The listing builds one solid part. Answer for the finished solid, in the listing's coordinates (mm). A direction names the side the tool comes from. Round coordinates to 2 decimals unless told otherwise and drop trailing zeros. Order: outer loops, then holes, each group sorted by start corner. A loop starts at its lowest first (then second) coordinate and runs counter-clockwise, first axis right, second up. Notation, with made-up numbers: (56.5, 55) - (111.5, 55) arc R13 ccw to (111.5, 65) - close; hole circle Ø4 at (68.25, 72.5). An arc over 180 degrees is marked (long way). Write item = value, one per line.
from build123d import *

# Parameters (mm, degrees)
BOSS_EXTRUDE1_DEPTH = 3.175


with BuildPart() as part:
    # Sketch1 → Boss-Extrude1 (new, symmetric)
    with BuildSketch(Plane.XY):
        with BuildLine():
            Line((-54.61, -57.15), (54.61, -57.15))
            ThreePointArc((54.61, -57.15), (56.406051224, -56.406051224), (57.15, -54.61))
            Line((57.15, -54.61), (57.15, 54.61))
            ThreePointArc((57.15, 54.61), (56.406051224, 56.406051224), (54.61, 57.15))
            Line((54.61, 57.15), (-54.61, 57.15))
            ThreePointArc((-54.61, 57.15), (-56.406051224, 56.406051224), (-57.15, 54.61))
            Line((-57.15, 54.61), (-57.15, -54.61))
            ThreePointArc((-57.15, -54.61), (-56.406051224, -56.406051224), (-54.61, -57.15))
        make_face()
        with BuildLine():
            Line((-45.72, -48.26), (11.649731947, -48.26))
            Line((11.649731947, -48.26), (45.72, -48.26))
            ThreePointArc((45.72, -48.26), (47.516051224, -47.516051224), (48.26, -45.72))
            Line((48.26, -45.72), (48.26, -17.513600374))
            Line((48.26, -17.513600374), (48.26, 45.72))
            ThreePointArc((48.26, 45.72), (47.516051224, 47.516051224), (45.72, 48.26))
            Line((45.72, 48.26), (12.317525133, 48.26))
            Line((12.317525133, 48.26), (-45.9238932, 48.26))
            ThreePointArc((-45.9238932, 48.26), (-46.572550677, 48.344222429), (-47.178191218, 48.591304348))
            ThreePointArc((-47.178191218, 48.591304348), (-54.010842502, 46.063523076), (-50.35826087, 39.760075674))
            ThreePointArc((-50.35826087, 39.760075674), (-48.854027571, 38.891201551), (-48.26, 37.2587827))
            Line((-48.26, 37.2587827), (-48.26, -0.752095073))
            Line((-48.26, -0.752095073), (-48.26, -45.72))
            ThreePointArc((-48.26, -45.72), (-47.516051224, -47.516051224), (-45.72, -48.26))
        make_face(mode=Mode.SUBTRACT)
    extrude(amount=BOSS_EXTRUDE1_DEPTH, both=True)


solid = part.part
Q1. Determine the mould class of faces 3 (the face through (-47.536, -47.496, 0.044)), 4 (the face through (-1, -57.15, 0)), 5 (the face through (-56.426, -56.386, 0.044)) for opening direction X: released by +X, released by -X, zero draft, split by the parting line, or undercut.
Model answer:
face_3 = undercut
face_4 = zero draft
face_5 = released by -X
Q2. Section A-A on x = -30.5 is taken. Determine the outline of the cut face in (y, z) (3 decimals), then the cut area to 3 significant figures.
Model answer:
outline = (-57.15, -3.175) - (-48.26, -3.175) - (-48.26, 3.175) - (-57.15, 3.175) - close; (48.26, -3.175) - (57.15, -3.175) - (57.15, 3.175) - (48.26, 3.175) - close
area = 113 mm^2
Q3. Find the intervals of material crossed by line 1 (X direction, y = 44.45, z = -1.5); line 2 (X direction, y = -17.5, z = -1), in increasing order. Write a range as from..to.
Model answer:
line_1 = -57.15..-54.29, 48.26..57.15
line_2 = -57.15..-48.26, 48.26..57.15
Q4. For faces 1 (the face through (-1, -48.26, 0)), 2 (the face through (56.386, -56.426, 0.044)), determine the directions among +Z, -Z, +X, -X, +Y, -Y from which every point of the face is accessible in a straight line to the end or side of a thin tool.
Model answer:
face_1 = +Z, -Z
face_2 = +Z, -Z, +X, -Y
